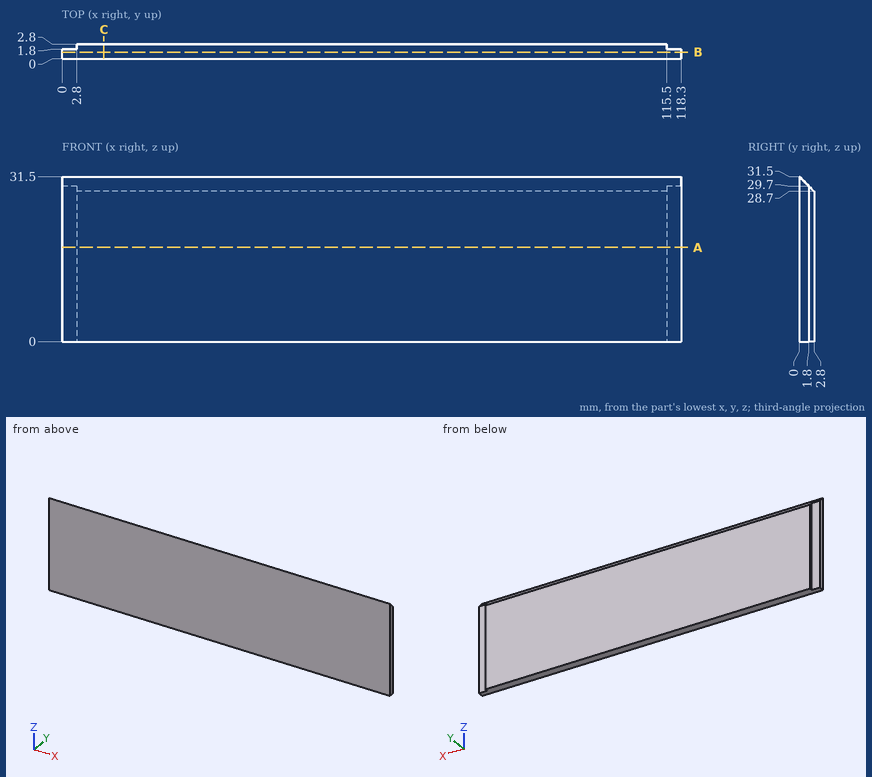
Drawing for the job (mm, zero at the part's lowest x, y, z). Give positions to 0.01 mm unless a question says otherwise; leave off trailing zeros. Loops run counter-clockwise (first coordinate to the right, second up) from the corner with the lowest first, then second, coordinate; pieces in that order, holes last. Notation, with made-up numbers: (6.5, 6) - (27.5, 6) arc R13 ccw to (27.5, 10) - close; hole circle Ø9 at (2.25, -38.75). An arc over 180 degrees is marked (long way). Write item = value, one per line. Start each with the question number.
1) Band-saw the part on A-A on z = 18. Give the cut face in (x, y), plus the area to 3 significant figures.
2) Probe probe 1 along X at (y, z) = (2.6, 17.5); probe 2 along Y at (x, z) = (77, 30); probe 3 along Z at (x, y) = (51, 0.2). List the from-to ranges inside material, lowest first. Write a range as from..to.
3) Band-saw the part on C-C on x = 8. Give the cut face in (y, z).
4) Band-saw the part on B-B on y = 1.25. Give the cut face in (x, z).
5) Drop a flat-ended pin along its axis: pin 1 Ø0.8 at (x, z) = (1, 14.5) entering from +Y. Give the stop position or say it passes through.
Final values:
q1.outline = (0, 0) - (118.3, 0) - (118.3, 1.8) - (115.5, 1.8) - (115.5, 2.8) - (2.8, 2.8) - (2.8, 1.8) - (0, 1.8) - close
q1.area = 326 mm²
q2.probe_1 = 2.8..115.5
q2.probe_2 = 0..1.5
q2.probe_3 = 0..31.3
q3.outline = (0, 0) - (2.8, 0) - (2.8, 28.7) - (0, 31.5) - close
q4.outline = (0, 0) - (118.3, 0) - (118.3, 30.25) - (0, 30.25) - close
q5.pin_1 = 1.8
